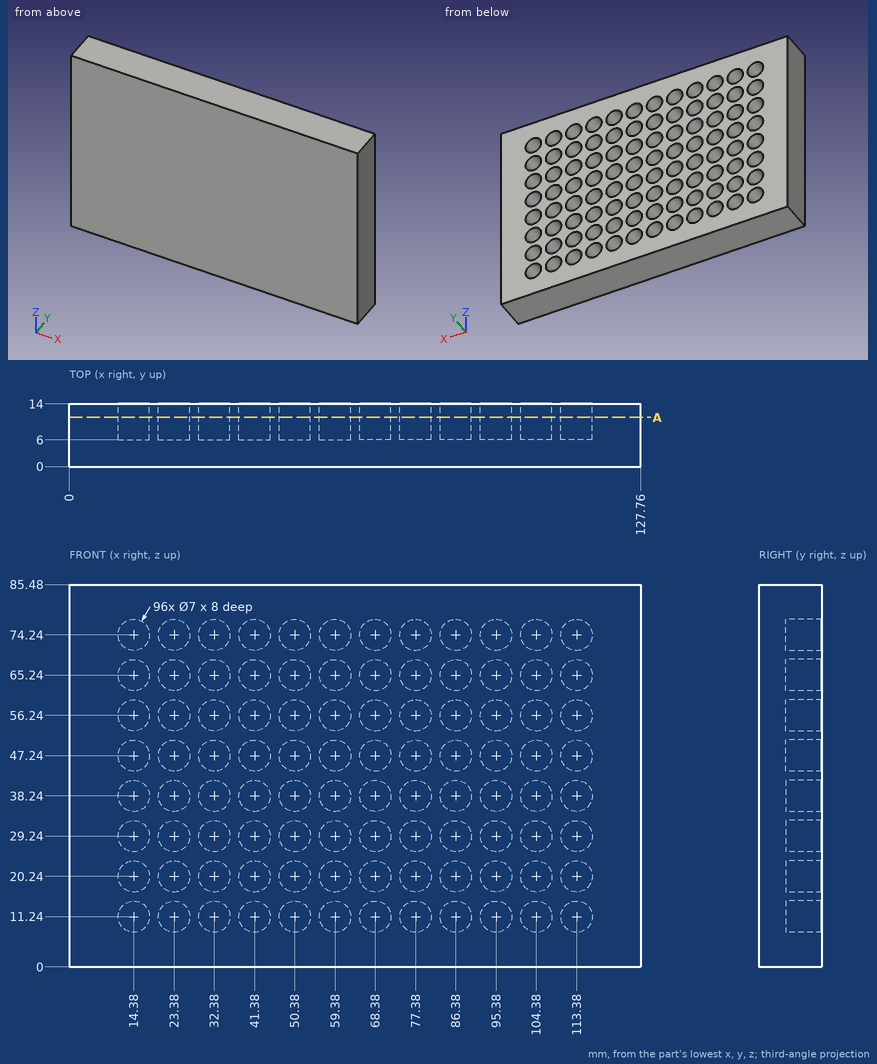
Design review of the part shown in the three views and the two pictorial views. Dimensions are in mm from the part's minimum x, y and z. Coordinates: 2 decimals unless noted, no trailing zeros. Put each result on its own line as item: value. Start each with the question number.
Q1. Wall thickness on line 1 (Y direction, x = 12, z = 75.5): over which ranges is the line inside the solid? List them lowest first.
Q2. Add section A-A (y = 11). Count the separate pieces of the cut face and the enclosed holes in it, and give its area (3 significant figures).
Q3. Clearance check with a flat-ended pin moving along its axis: pin 1 (3.5 mm diameter, centred on x = 113, z = 28, fed in from +Y). State where the tip first meets the part, or that it passes through.
Answers:
1. line 1: y = 0 to 6
2. separate pieces: 1
2. enclosed holes: 96
2. area: 7,230 mm^2
3. pin 1: stops at y = 6
